Input: part model. Units: mm. Frame: model coordinates. A direction names the side the tool comes from. Give positions to 0.01 mm unless a question says otherwise; leave off trailing zeros. Order: outer loops, then holes, each group sorted by start corner. A loop starts at its lowest first (then second) coordinate and runs counter-clockwise, first axis right, second up. Notation, with made-up numbers: (52, -23) - (77, -23) arc R25 cw to (77, 10) - close; hole circle Ø6 at (-1, 61.25). An arc over 180 degrees is marked (long way). Answer in a Markdown table with one row per item. Add a question column.
from build123d import *

# Parameters (mm, degrees)
F1_DEPTH = 3


# Not quite as in the source:
# - a feature names something its author has since deleted; it is built from what else it names


with BuildPart() as f1:
    # F0 (on Right) → F1 (new body)
    with BuildSketch(Plane.YZ):
        Polygon((-1.8767494946, 26.7287779992), (-7.8767494946, 26.7287779992), (-7.8767494946, 24.7287779992), (-6.3767494946, 24.7287779992), (-6.3767494946, 22.2287779992), (-7.8767494946, 22.2287779992), (-7.8767494946, 11.7737779992), (-10.8767494946, 11.7737779992), (-10.8767494946, 6.7737779992), (-7.8767494946, 6.7737779992), (-7.8767494946, 3.7737779992), (7.1232505054, 26.7287779992), (3.1232505054, 26.7287779992), (3.1232505054, 29.7287779992), (-1.8767494946, 29.7287779992), align=None)
    extrude(amount=F1_DEPTH)


solid = f1.part
Q1. Access query for faces 5 (the flat face through (1, 3.123, 28)), 6 (the flat face through (1, -6.377, 23)), 7 (the flat face through (1, -7.877, 5)), 8 (the flat face through (1, -9, 11.774)). Directions: +Z, -Z, +X, -X, +Y, -Y. A direction counts if a zero-diameter tool reaches every point of the face in a straight line with its end or side. Return the directions, or none.
Q2. Contact query for flat-ended pins moving along their axis: P1, Ø1, axis at x = 2.5, y = 4, coming from the +Z side; P2, Ø1.5, axis at x = 2, z = 28, coming from the -Y side; P3, Ø0.9, axis at x = 2, z = 5.5, coming from the -Y side. Output: stop coordinate, or through.
Q3. Pull-direction query (Z, two-part tool) for faces 1 (the flat face through (1, -9, 6.774)), 2 (the flat face through (1, 5, 26.729)), 3 (the flat face through (1, -7, 22.229)), 4 (the flat face through (0, -2, 20)); classes: +Z half, -Z half, draft (parallel to the pull), parting line (faces both ways), or undercut.
Q4. Section A-A, the plane x = 2.1. Return loops of the section in (y, z).
Q5. Line query: probe 1 along Y at (x, z) = (1.2, 27.25); probe 2 along Z at (x, y) = (1.8, -8.5); probe 3 along Z at (x, y) = (2.7, 2.5). Output: solid intervals per line, ascending.
Q6. Section C-C, the plane z = 27.25. Return loops of the section in (x, y).
Q7. Section B-B, the plane y = -6.75. Return loops of the section in (x, z).
Q8. Section D-D, the plane y = -9. Return loops of the section in (x, z), then the cut area to 3 significant figures.
Computed:
| question | item | result |
|---|---|---|
| 1 | face 5 | +Z, +X, -X, +Y |
| 1 | face 6 | +X, -X, -Y |
| 1 | face 7 | -Z, +X, -X, -Y |
| 1 | face 8 | +Z, +X, -X, -Y |
| 2 | P1 | stops at z = 26.73 |
| 2 | P2 | stops at y = -1.88 |
| 2 | P3 | stops at y = -7.88 |
| 3 | face 1 | -Z half |
| 3 | face 2 | +Z half |
| 3 | face 3 | undercut |
| 3 | face 4 | draft |
| 4 | outline | (-10.88, 6.77) - (-7.88, 6.77) - (-7.88, 3.77) - (7.12, 26.73) - (3.12, 26.73) - (3.12, 29.73) - (-1.88, 29.73) - (-1.88, 26.73) - (-7.88, 26.73) - (-7.88, 24.73) - (-6.38, 24.73) - (-6.38, 22.23) - (-7.88, 22.23) - (-7.88, 11.77) - (-10.88, 11.77) - close |
| 5 | probe 1 | y = -1.88 to 3.12 |
| 5 | probe 2 | z = 6.77 to 11.77 |
| 5 | probe 3 | z = 19.65 to 29.73 |
| 6 | outline | (0, -1.88) - (3, -1.88) - (3, 3.12) - (0, 3.12) - close |
| 7 | outline | (0, 5.5) - (3, 5.5) - (3, 22.23) - (0, 22.23) - close; (0, 24.73) - (3, 24.73) - (3, 26.73) - (0, 26.73) - close |
| 8 | outline | (0, 6.77) - (3, 6.77) - (3, 11.77) - (0, 11.77) - close |
| 8 | area | 15.0 mm^2 |
